Input: part model. Units: mm. Frame: model coordinates. Face numbers are marked on the shaded views. A direction names the side the tool comes from. Give positions to 0.01 mm unless a question says otherwise; leave off trailing zeros. Loops run counter-clockwise (first coordinate to the right, second up) from the corner with the lowest first, then second, coordinate; pieces in that order, holes last. Notation, with made-up numbers: M -40,69.25 L 15,69.25 A24 cw 15,94.25 Z; hole C 27,57 d11. An arc over 180 degrees is marked long. One line per item, written item: value. Start each with the question number.
(1) Pull-direction query (Y, two-part tool) for the marked faces 1, 2 and 3; classes: released by +Y, released by -Y, zero draft, split by the parting line, or undercut.
(2) Section A-A on z = 7.75. Output: boundary loops of the cut face in (x, y).
(3) Section B-B on x = -32.4. Output: boundary loops of the cut face in (y, z).
(4) Section C-C on x = -7.4. Output: boundary loops of the cut face in (y, z).
(5) Pin query (flat end, axial travel): P1, Ø5.5, axis at y = 1.5, z = 4.5, coming from the -X side; P2, Ø3, axis at x = 43.6, z = 2.34, coming from the -Y side; P3, Ø1.5, axis at y = 4.5, z = 5.5, coming from the +X side; P4, Ø2.5, axis at x = -32.5, z = -0.5, coming from the -Y side. Return the tip coordinate at first contact, or that it passes through.
(6) Section D-D on y = -7.5. Output: boundary loops of the cut face in (x, z).
(7) Access query for the marked faces 4 and 5. Directions: +Z, -Z, +X, -X, +Y, -Y. A direction counts if a zero-diameter tool reaches every point of the face in a straight line with its end or side. Return the directions, or none.
(8) Ray query, line 1 along Y through (x, z) = (25, 2.5); line 2 along X through (y, z) = (5.25, 7); line 3 along X through (y, z) = (9.5, 2.5). Return the intervals inside material, ascending. Write a range as from..to.
Solid Edge part; units mm, degrees
sketch "Sketch1" plane through (0, 0, 0) normal (0, 0, 1) x (1, 0, 0)
  line L0 (-29.4, -11) -> (65.6, -11)
  line L1 (65.6, -11) -> (65.6, -3)
  line L2 (71.6, -3) -> (65.6, -3)
  line L3 (71.6, -3) -> (71.6, 3)
  line L4 (71.6, 3) -> (65.6, 3)
  line L5 (65.6, 3) -> (65.6, 11)
  line L6 (65.6, 11) -> (-29.4, 11)
  line L7 (-29.4, 3) -> (-29.4, 11)
  line L8 (-35.4, 3) -> (-29.4, 3)
  line L9 (-35.4, 3) -> (-35.4, -3)
  line L10 (-29.4, -3) -> (-35.4, -3)
  line L11 (-29.4, -11) -> (-29.4, -3)
  circle A0 centre (68.6, 0) radius 1.5
  circle A1 centre (-32.4, 0) radius 1.5
  line L12 (1.5343, -4) -> (9.5343, 4)
  line L13 (9.5343, 4) -> (2.6657, 4)
  line L14 (-5.3343, -4) -> (2.6657, 4)
  line L15 (-5.3343, -4) -> (1.5343, -4)
  line L16 (-6.4657, -4) -> (1.5343, 4)
  line L17 (1.5343, 4) -> (-5.3343, 4)
  line L18 (-13.3343, -4) -> (-5.3343, 4)
  line L19 (-13.3343, -4) -> (-6.4657, -4)
  line L20 (-21.9, -3.4343) -> (-14.4657, 4)
  line L21 (-14.4657, 4) -> (-21.9, 4)
  line L22 (-21.9, 4) -> (-21.9, -3.4343)
  line L23 (57.5343, 4) -> (50.6657, 4)
  line L24 (42.6657, -4) -> (50.6657, 4)
  line L25 (42.6657, -4) -> (49.5343, -4)
  line L26 (49.5343, -4) -> (57.5343, 4)
  line L27 (-14.4657, -4) -> (-6.4657, 4)
  line L28 (-6.4657, 4) -> (-13.3343, 4)
  line L29 (-21.3343, -4) -> (-13.3343, 4)
  line L30 (-21.3343, -4) -> (-14.4657, -4)
  line L31 (17.5343, -4) -> (25.5343, 4)
  line L32 (25.5343, 4) -> (18.6657, 4)
  line L33 (10.6657, -4) -> (18.6657, 4)
  line L34 (10.6657, -4) -> (17.5343, -4)
  line L35 (34.6657, -4) -> (42.6657, 4)
  line L36 (49.5343, 4) -> (42.6657, 4)
  line L37 (41.5343, -4) -> (49.5343, 4)
  line L38 (34.6657, -4) -> (41.5343, -4)
  line L39 (33.5343, -4) -> (41.5343, 4)
  line L40 (41.5343, 4) -> (34.6657, 4)
  line L41 (26.6657, -4) -> (34.6657, 4)
  line L42 (26.6657, -4) -> (33.5343, -4)
  line L43 (9.5343, -4) -> (17.5343, 4)
  line L44 (17.5343, 4) -> (10.6657, 4)
  line L45 (2.6657, -4) -> (10.6657, 4)
  line L46 (2.6657, -4) -> (9.5343, -4)
  line L47 (25.5343, -4) -> (33.5343, 4)
  line L48 (33.5343, 4) -> (26.6657, 4)
  line L49 (18.6657, -4) -> (26.6657, 4)
  line L50 (18.6657, -4) -> (25.5343, -4)
  line L51 (50.6657, -4) -> (58.1, -4)
  line L52 (58.1, 3.4343) -> (58.1, -4)
  line L53 (50.6657, -4) -> (58.1, 3.4343)
extrude "Protrusion1" add sketch "Sketch1" against normal blind 2
sketch "Sketch2" plane through (0, 0, 0) normal (0, 0, 1) x (1, 0, 0)
  line L0 (-27.4, -9) -> (63.6, -9)
  line L1 (63.6, -9) -> (63.6, 9)
  line L2 (63.6, 9) -> (-27.4, 9)
  line L3 (-27.4, -9) -> (-27.4, 9)
  line L4 (65.6, 11) -> (-29.4, 11)
  line L5 (-29.4, 3) -> (-29.4, 11)
  line L6 (-29.4, -3) -> (-29.4, 3)
  line L7 (-29.4, -11) -> (-29.4, -3)
  line L8 (-29.4, -11) -> (65.6, -11)
  line L9 (65.6, -11) -> (65.6, -3)
  line L10 (65.6, -3) -> (65.6, 3)
  line L11 (65.6, 3) -> (65.6, 11)
extrude "ExtrudedProtrusion_2" add sketch "Sketch2" along normal blind 10
fillet "Round_2" radius 1 4 edges at (71.6, -3, -1) (71.6, 3, -1) (-35.4, -3, -1) (-35.4, 3, -1)
sketch "Sketch3" plane through (0, -11, 5.5) normal (0, -1, 0) x (1, 0, 0)
  circle A0 centre (-7.4, -3.1597) radius 1.6
  circle A1 centre (43.6, -3.1597) radius 1.6
extrude "ExtrudedCutout_3" cut sketch "Sketch3" against normal blind 26
chamfer "Chamfer_5" distance 1 angle 45 2 edges at (-29.4, 0, 0) (65.6, 0, 0)
fillet "Round_7" radius 1 4 edges at (-29.4, 0, 10) (18.1, -11, 10) (18.1, 11, 10) (65.6, 0, 10)
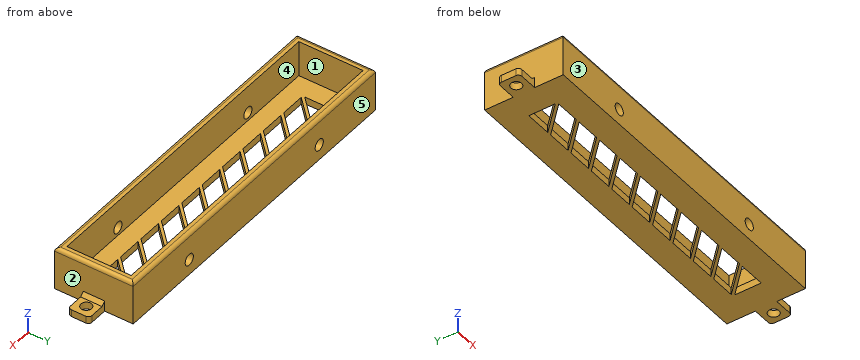
Output values:
1. face 1: undercut
1. face 2: zero draft
1. face 3: released by -Y
2. outline: M -29.4,-11 L 65.6,-11 L 65.6,11 L -29.4,11 Z; hole M -27.4,-9 L 63.6,-9 L 63.6,9 L -27.4,9 Z
3. outline: M -3,-2 L -1.5,-2 L -1.5,0 L -3,0 Z; M 1.5,-2 L 3,-2 L 3,0 L 1.5,0 Z
4. outline: M -11,-2 L -4,-2 L -4,0 L -9,0 L -9,0.74 L -11,0.74 Z; M -11,3.94 L -9,3.94 L -9,10 L -10,10 A1 ccw -11,9 Z; M 1.93,-2 L 3.07,-2 L 3.07,0 L 1.93,0 Z; M 4,-2 L 11,-2 L 11,0.74 L 9,0.74 L 9,0 L 4,0 Z; M 9,3.94 L 11,3.94 L 11,9 A1 ccw 10,10 L 9,10 Z
5. P1: stops at x = -29.4
5. P2: passes through
5. P3: stops at x = 65.6
5. P4: stops at y = -3
6. outline: M -29.4,-2 L 65.6,-2 L 65.6,9 A1 ccw 64.6,10 L 63.6,10 L 63.6,0 L -27.4,0 L -27.4,10 L -28.4,10 A1 ccw -29.4,9 Z
7. face 4: +Z
7. face 5: +Z, -Z, +X, -X, +Y
8. line 1: y = -11..-9, 9..11
8. line 2: x = -29.4..-27.4, 63.6..65.6
8. line 3: x = -29.4..-8.99, -5.81..42.01, 45.19..65.6
